```python
from build123d import *

# Parameters (mm, degrees)
SKETCH1_R           = 2.25
BOSS_EXTRUDE1_DEPTH = 5
SKETCH2_R           = 2.25
CUT_EXTRUDE1_DEPTH  = 72.702510416
SKETCH3_W           = 10
SKETCH3_H           = 16
CUT_EXTRUDE2_DEPTH  = 69.689518851
CHAMFER1_SIZE       = 3


with BuildPart() as part:
    # Sketch1 → Boss-Extrude1 (new, symmetric)
    with BuildSketch(Plane(origin=(0, 0, 0), x_dir=(0, 0, -1), z_dir=(1, 0, 0))):
        with BuildLine():
            Line((-20, -56), (38.5, -56))
            Line((38.5, -56), (38.5, 6))
            Line((38.5, 6), (0, 6))
            ThreePointArc((0, 6), (-6, 0), (0, -6))
            Line((0, -6), (18.5, -6))
            Line((18.5, -6), (18.5, -44))
            Line((18.5, -44), (-20, -44))
            ThreePointArc((-20, -44), (-26, -50), (-20, -56))
        make_face()
        Circle(SKETCH1_R, mode=Mode.SUBTRACT)
        with Locations((0, -50)):
            Circle(SKETCH1_R, mode=Mode.SUBTRACT)
        with Locations((-20, -50)):
            Circle(SKETCH1_R, mode=Mode.SUBTRACT)
    extrude(amount=BOSS_EXTRUDE1_DEPTH, both=True)

    # Sketch2 → Cut-Extrude1 (cut, through all)
    with BuildSketch(Plane.XY.offset(-18.5)):
        with Locations((0, -16.1)):
            Circle(SKETCH2_R)
        with Locations((0, -36.1)):
            Circle(SKETCH2_R)
    extrude(amount=-CUT_EXTRUDE1_DEPTH, mode=Mode.SUBTRACT)

    # Sketch3 → Cut-Extrude2 (cut, through all)
    with BuildSketch(Plane(origin=(5, 0, 0), x_dir=(0, 0, -1), z_dir=(1, 0, 0))):
        with Locations((33.5, -2)):
            Rectangle(SKETCH3_W, SKETCH3_H)
    extrude(amount=-CUT_EXTRUDE2_DEPTH, mode=Mode.SUBTRACT)

    # Chamfer1
    chamfer1_edges = [part.edges().sort_by_distance(p)[0] for p in [
        (0, -44, -18.5),
        (0, -6, -18.5),
        (0, -56, -38.5),
        (0, -10, -38.5),
        (0, 6, -28.5),
    ]]
    chamfer(chamfer1_edges, length=CHAMFER1_SIZE)


solid = part.part
```
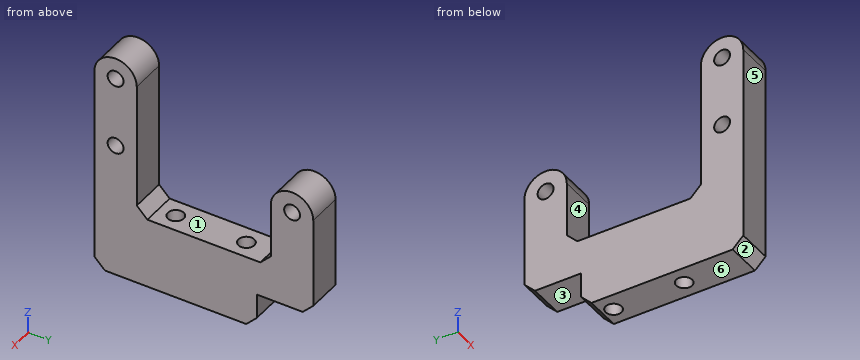
Source: CAD feature listing. Evaluate the final solid. Frame: model axes, mm. Face numbers are marked on the shaded views. A direction names the side the tool comes from. Round coordinates to 2 decimals unless told otherwise and drop trailing zeros. Loops run counter-clockwise (first coordinate to the right, second up) from the corner with the lowest first, then second, coordinate; pieces in that order, holes last. Notation, with made-up numbers: M 84.5,-4.75 L 139.5,-4.75 A22 ccw 139.5,16.25 Z; hole C -5,5 d9. An arc over 180 degrees is marked long. Use a Markdown table: item, result. Add a question column.
1. Cut plane D-D, the plane x = -3.5. Output: boundary loops of the cut face in (y, z).
2. Cut plane A-A, the plane x = 0. Output: boundary loops of the cut face in (y, z).
3. Ray query, line 1 along Y through (x, z) = (-0.25, 0); line 2 along Y through (x, z) = (0, -32.5); line 3 along Y through (x, z) = (1, -5). Return the intervals inside material, ascending. Write a range as [from, to].
4. Cut plane B-B, the plane y = 0. Output: boundary loops of the cut face in (x, z), and give its area (3 significant figures).
5. Contact query for flat-ended pins moving along their axis: pin 1 (12 mm diameter, centred on y = -39.5, z = 6.5, fed in from -X); pin 2 (3.5 mm diameter, centred on y = 0, z = 0, fed in from -X); pin 3 (3.5 mm diameter, centred on x = -2, z = -31.5, fed in from +Y). Output: stop coordinate, or through.
6. Set-up query: the marked faces 1, 2 and 3. Return all of +Z, -Z, +X, -X, +Y, -Y with unobstructed straight access to the full face (end or side cutting, diameter ignored); none if empty.
7. Pull-direction query (Y, two-part tool) for the marked faces 4, 5 and 6; classes: +Y half, -Y half, draft (parallel to the pull), parting line (faces both ways), or undercut.
8. Cut plane C-C, the plane y = -50. Output: boundary loops of the cut face in (x, z).
Solution:
| question | item | result |
|---|---|---|
| 1 | outline | M -56,-35.5 L -53,-38.5 L -13,-38.5 L -10,-35.5 L -10,-28.5 L 3,-28.5 L 6,-25.5 L 6,0 A6 ccw -6,0 L -6,-15.5 L -9,-18.5 L -41,-18.5 L -44,-15.5 L -44,20 A6 ccw -56,20 Z; hole C -50,0 d4.5; hole C -50,20 d4.5; hole C 0,0 d4.5 |
| 2 | outline | M -56,-35.5 L -53,-38.5 L -38.35,-38.5 L -38.35,-18.5 L -41,-18.5 L -44,-15.5 L -44,20 A6 ccw -56,20 Z; M -33.85,-38.5 L -18.35,-38.5 L -18.35,-18.5 L -33.85,-18.5 Z; M -13.85,-38.5 L -13,-38.5 L -10,-35.5 L -10,-28.5 L 3,-28.5 L 6,-25.5 L 6,0 A6 ccw -6,0 L -6,-15.5 L -9,-18.5 L -13.85,-18.5 Z; hole C -50,0 d4.5; hole C -50,20 d4.5; hole C 0,0 d4.5 |
| 3 | line 1 | y = [-56, -52.25], [-47.75, -44], [-6, -2.25], [2.25, 6] |
| 3 | line 2 | y = [-56, -38.35], [-33.85, -18.35], [-13.85, -10] |
| 3 | line 3 | y = [-56, -44], [-6, 6] |
| 4 | outline | M -5,-28.5 L 5,-28.5 L 5,-2.25 L -5,-2.25 Z; M -5,2.25 L 5,2.25 L 5,6 L -5,6 Z |
| 4 | area | 300 mm2 |
| 5 | pin 1 | stops at x = -5 |
| 5 | pin 2 | passes through |
| 5 | pin 3 | stops at y = -10 |
| 6 | face 1 | +Z, +X, -X |
| 6 | face 2 | -Z, +X, -X, -Y |
| 6 | face 3 | -Z, +X, -X, +Y |
| 7 | face 4 | undercut |
| 7 | face 5 | -Y half |
| 7 | face 6 | draft |
| 8 | outline | M -5,-38.5 L 5,-38.5 L 5,-2.25 L -5,-2.25 Z; M -5,2.25 L 5,2.25 L 5,17.75 L -5,17.75 Z; M -5,22.25 L 5,22.25 L 5,26 L -5,26 Z |
